Source: CAD feature listing. Evaluate the final solid. Frame: model axes, mm. Face numbers are marked on the shaded views. A direction names the side the tool comes from. Give positions to 0.01 mm unless a question says otherwise; leave off trailing zeros. Loops run counter-clockwise (first coordinate to the right, second up) from the corner with the lowest first, then second, coordinate; pieces in that order, holes last.
```python
from build123d import *

# Parameters (mm, degrees)
SKETCH1_R               = 40
BOSS_EXTRUDE1_DEPTH     = 74.5
SKETCH3_R               = 40
SKETCH3_R_2             = 25
CUT_EXTRUDE1_DEPTH      = 21
CUT_EXTRUDE2_DEPTH      = 22
CUT_EXTRUDE2_DEPTH_BACK = 22
SKETCH2_R               = 40
SKETCH2_R_2             = 37.5
CUT_EXTRUDE4_DEPTH      = 160.376911753
FILLET1_R               = 2
CUT_EXTRUDE5_DEPTH      = 160.376911753


with BuildPart() as part:
    # Sketch1 → Boss-Extrude1 (new, symmetric)
    with BuildSketch(Plane(origin=(0, 0, 0), x_dir=(1, 0, 0), z_dir=(0, 1, 0))):
        with Locations(Location((0, 0, 0), (0, 0, 270))):
            Circle(SKETCH1_R)
    extrude(amount=BOSS_EXTRUDE1_DEPTH, both=True)

    # Sketch3 → Cut-Extrude1 (cut)
    with BuildSketch(Plane(origin=(0, 74.5, 0), x_dir=(1, 0, 0), z_dir=(0, 1, 0))):
        with Locations(Location((0, 0, 0), (0, 0, 270))):
            Circle(SKETCH3_R)
        with Locations(Location((0, 0, 0), (0, 0, 270))):
            Circle(SKETCH3_R_2, mode=Mode.SUBTRACT)
    cut_extrude1 = extrude(amount=-CUT_EXTRUDE1_DEPTH, mode=Mode.SUBTRACT)

    # Mirror1: Cut-Extrude1 across plane
    add(cut_extrude1.mirror(Plane.ZX), mode=Mode.SUBTRACT)

    # Sketch2 → Cut-Extrude2 (cut, two sides: drawn at the far end of the back side and taken through both)
    with BuildSketch(Plane(origin=(0, 0, 0), x_dir=(1, 0, 0), z_dir=(0, 1, 0)).offset(-CUT_EXTRUDE2_DEPTH_BACK)):
        with Locations(Location((0, 0, 0), (0, 0, 270))):
            Circle(SKETCH2_R)
        with Locations(Location((0, 0, 0), (0, 0, 90))):
            Circle(SKETCH2_R_2, mode=Mode.SUBTRACT)
    extrude(amount=CUT_EXTRUDE2_DEPTH + CUT_EXTRUDE2_DEPTH_BACK, mode=Mode.SUBTRACT)

    # Sketch5 → Cut-Extrude4 (cut, through all)
    with BuildSketch(Plane(origin=(0, 74.5, 0), x_dir=(1, 0, 0), z_dir=(0, 1, 0))):
        with BuildLine():
            Line((-12, 13), (12, 13))
            ThreePointArc((12, 13), (15, 10), (12, 7))
            Line((12, 7), (-12, 7))
            ThreePointArc((-12, 7), (-15, 10), (-12, 13))
        make_face()
    extrude(amount=-CUT_EXTRUDE4_DEPTH, mode=Mode.SUBTRACT)

    # Fillet1
    fillet1_edges = [part.edges().sort_by_distance(p)[0] for p in [
        (0, -53.5, -25),
        (0, 53.5, -25),
    ]]
    fillet(fillet1_edges, radius=FILLET1_R)

    # Sketch7 → Revolve2 (revolve)
    with BuildSketch(Plane(origin=(0, 0, 0), x_dir=(0, 0, -1), z_dir=(1, 0, 0))):
        Polygon((40, 22), (37.5, 19.5), (37.5, 22), align=None)
    revolve2 = revolve(axis=Axis((0, 103.881416882, 0), (0, -1, 0)))

    # Mirror2: Revolve2 across plane
    add(revolve2.mirror(Plane.ZX))

    # Sketch4 → Cut-Extrude5 (cut, through all)
    with BuildSketch(Plane(origin=(0, 74.5, 0), x_dir=(1, 0, 0), z_dir=(0, 1, 0))):
        with BuildLine():
            Line((0, 0), (0, 40))
            ThreePointArc((0, 40), (28.284271247, 28.284271247), (40, 0))
            Line((40, 0), (0, 0))
        make_face()
    extrude(amount=-CUT_EXTRUDE5_DEPTH, mode=Mode.SUBTRACT)


solid = part.part
```
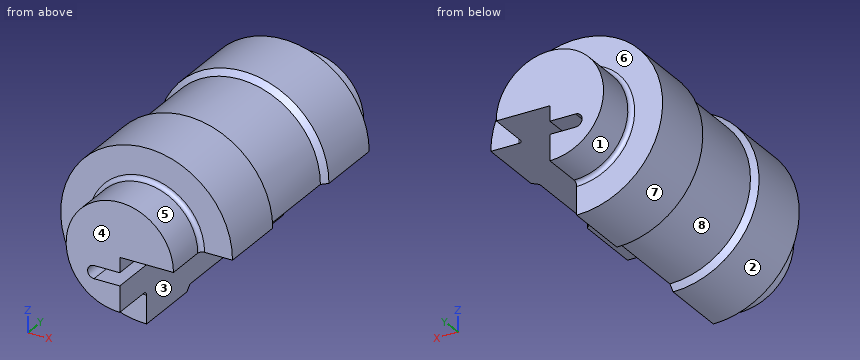
(1) First-contact query: pin 1 (12 mm diameter, centred on x = 26, z = 31.5, fed in from +Y); pin 2 (21.5 mm diameter, centred on y = -23, z = -30, fed in from +X); pin 3 (1.5 mm diameter, centred on x = -23, y = -55.5, fed in from -Z). Flat tips, straight axial feed; report the tip coordinate or a pass-through.
A:
pin 1: stops at y = 53.5
pin 2: stops at x = 0
pin 3: stops at z = -11.4
(2) Reachability of the marked faces 1, 2, 3, 4 and 5 from +Z, -Z, +X, -X, +Y, -Y: full face, straight path, thin tool, end or side. Return the list, or none.
A:
face 1: +Y
face 2: +Y, -Y
face 3: -Z, +X, +Y, -Y
face 4: +Z, -Z, +X, -X, -Y
face 5: -Y
(3) Section A-A, the plane y = -59. Return the cut outline in (x, z).
A:
outline: (-12, -13) arc R3 cw to (-12, -7) - (0, -7) - (0, 0) - (25, 0) arc R25 ccw (long way) to (0, -25) - (0, -13) - close
(4) Ray query, line 1 along Y through (x, z) = (30, 23); line 2 along X through (y, z) = (22.5, 14); line 3 along Y through (x, z) = (-3, 26.5). Return the intervals inside material, ascending.
A:
line 1: y = -53.5 to -19.8, 19.8 to 53.5
line 2: x = -37.47 to 37.47
line 3: y = -53.53 to 53.53
(5) Mould query, pull axis Y, two halves, no side actions, for the marked faces 6, 7 and 8. Classes: pulls with the +Y half, pulls with the -Y half, needs draft (parallel to the pull), parting line crosses it, or undercut.
A:
face 6: pulls with the +Y half
face 7: needs draft
face 8: undercut
